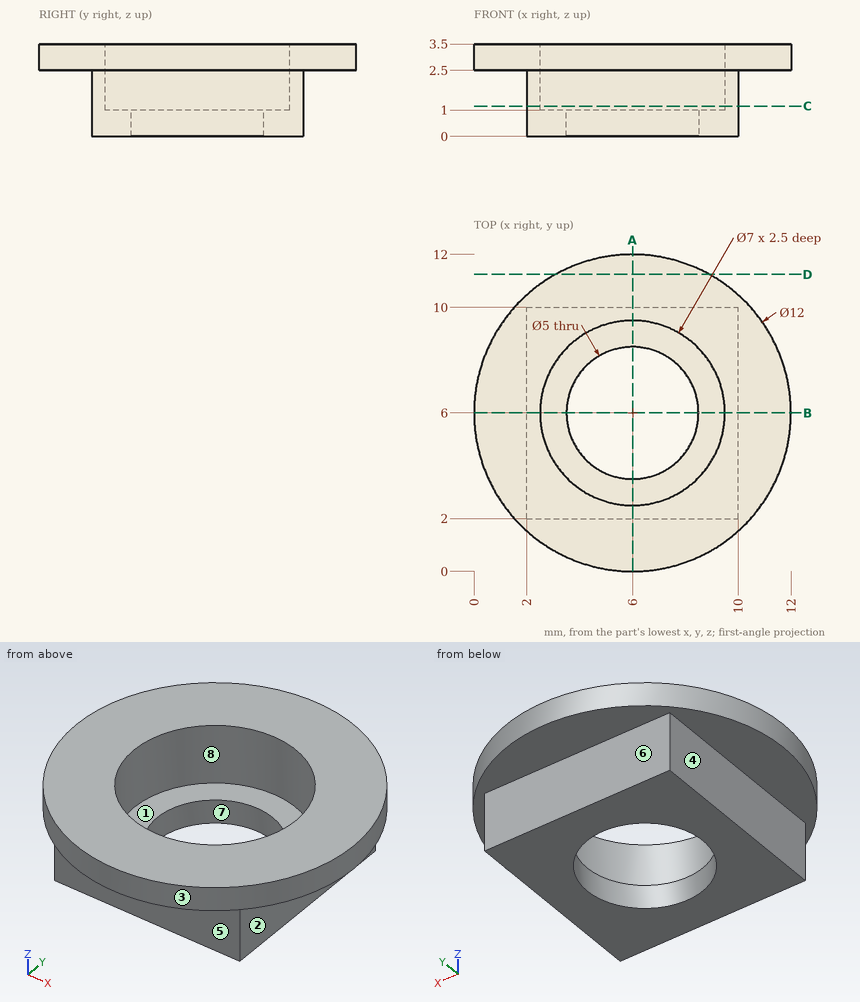
Job drawing, mm, ordinate dimensions from the low corner. One solid piece. A direction names the side the tool comes from. Coordinates: 2 decimals unless noted, no trailing zeros. Order: outer loops, then holes, each group sorted by start corner. A loop starts at its lowest first (then second) coordinate and runs counter-clockwise, first axis right, second up. Notation, with made-up numbers: (-30.5, 44) - (26.5, 44) arc R8 cw to (26.5, 59) - close; hole circle Ø4 at (86.25, 41.5). An arc over 180 degrees is marked (long way). Write each question's results on one line, items separated by ' | '. Start each with the question number.
Item 1: Flat gauge pins, fed straight in: pin 1 (2 mm diameter, centred on x = 7, y = 4.5, fed in from +Z); pin 2 (0.8 mm diameter, centred on y = 6, z = 0.5, fed in from +X); pin 3 (2 mm diameter, centred on x = 4.5, z = 2, fed in from -Y). Where does each tip first touch, or does it go through?
Item 2: Band-saw the part on A-A on x = 6. Write the cut outline in (y, z), and give its area (3 significant figures).
Item 3: Tool access for the marked faces 4, 5, 6, 7 and 8: list every direction of +Z, -Z, +X, -X, +Y, -Y with a clear straight run to the whole face (end or side of a thin tool).
Item 4: Band-saw the part on D-D on y = 11.25. Write the cut outline in (x, z).
Item 5: Wall check: probe 1 along Y at (x, z) = (6, 0.55); probe 2 along Y at (x, z) = (6, 1.05); probe 3 along Z at (x, y) = (4, 3.75). Give the ranges that are in metal, low to high. Write a range as [from, to].
Item 6: Mould opens along Y. For the marked faces 1, 2 and 3 say: released by +Y, released by -Y, zero draft, split by the parting line, or undercut.
Item 7: Band-saw the part on C-C on z = 1.15. Write the cut outline in (x, y), and give its area (3 significant figures).
Numbers:
1) pin 1: z = 1 | pin 2: x = 10 | pin 3: y = 0.03
2) outline: (0, 2.5) - (2, 2.5) - (2, 0) - (3.5, 0) - (3.5, 1) - (2.5, 1) - (2.5, 3.5) - (0, 3.5) - close; (8.5, 0) - (10, 0) - (10, 2.5) - (12, 2.5) - (12, 3.5) - (9.5, 3.5) - (9.5, 1) - (8.5, 1) - close | area: 9.50 mm^2
3) face 4: -Z, -X, +Y, -Y | face 5: -Z, +X, -X, -Y | face 6: -Z, +X, -X, +Y | face 7: +Z, -Z | face 8: +Z
4) outline: (3.1, 2.5) - (8.9, 2.5) - (8.9, 3.5) - (3.1, 3.5) - close
5) probe 1: [2, 3.5], [8.5, 10] | probe 2: [2, 2.5], [9.5, 10] | probe 3: [0, 1]
6) face 1: undercut | face 2: zero draft | face 3: split by the parting line
7) outline: (2, 2) - (10, 2) - (10, 10) - (2, 10) - close; hole circle Ø7 at (6, 6) | area: 25.5 mm^2
